from build123d import *

# Parameters (mm, degrees)
SKETCH1_W                      = 256.5
SKETCH1_H                      = 320
BASE_FLANGE1_DEPTH             = 0.9
EDGE_FLANGE1_STRIP_W           = 5.4
EDGE_FLANGE1_STRIP_H           = 0.9
EDGE_FLANGE1_STRIP_CUT_DEPTH   = 320
EDGE_FLANGE1_STRIP_2_W         = 5.4
EDGE_FLANGE1_STRIP_2_H         = 0.9
EDGE_FLANGE1_STRIP_CUT_2_DEPTH = 320
EDGE_FLANGE1_DEPTH             = 320
EDGE_FLANGE1_BEND_DEPTH        = 320
EDGE_FLANGE2_STRIP_W           = 5.4
EDGE_FLANGE2_STRIP_H           = 0.9
EDGE_FLANGE2_STRIP_CUT_DEPTH   = 320
EDGE_FLANGE2_DEPTH             = 320
CUT_EXTRUDE1_DEPTH             = 206.751482376


# Sheet-metal steps are written as plain solids
with BuildPart() as part:
    # Sketch1 → Base-Flange1 (new body)
    with BuildSketch(Plane.XY):
        Rectangle(SKETCH1_W, SKETCH1_H)
    extrude(amount=-BASE_FLANGE1_DEPTH)

    # Edge-Flange1 strip (across the edge) → Edge-Flange1 strip cut (cut)
    with BuildSketch(Plane(origin=(128.25, 160, -0.9), x_dir=(-1, 0, 0), z_dir=(0, -1, 0))):
        with Locations((-0.9, -0.45)):
            Rectangle(EDGE_FLANGE1_STRIP_W, EDGE_FLANGE1_STRIP_H)
    extrude(amount=EDGE_FLANGE1_STRIP_CUT_DEPTH, mode=Mode.SUBTRACT)

    # Edge-Flange1 strip 2 (across the edge) → Edge-Flange1 strip cut 2 (cut)
    with BuildSketch(Plane(origin=(-128.25, -160, -0.9), x_dir=(1, 0, 0), z_dir=(0, 1, 0))):
        with Locations((-0.9, -0.45)):
            Rectangle(EDGE_FLANGE1_STRIP_2_W, EDGE_FLANGE1_STRIP_2_H)
    extrude(amount=EDGE_FLANGE1_STRIP_CUT_2_DEPTH, mode=Mode.SUBTRACT)

    # Edge-Flange1 section (across the edge) → Edge-Flange1 (add)
    with BuildSketch(Plane(origin=(128.25, 160, -0.9), x_dir=(-1, 0, 0), z_dir=(0, -1, 0))):
        with BuildLine():
            Line((0, 0.9), (0, 15.1))
            Line((0, 15.1), (0.9, 15.1))
            Line((0.9, 15.1), (0.9, 0.9))
            ThreePointArc((0.9, 0.9), (1.163603897, 0.263603897), (1.8, 0))
            Line((1.8, 0), (1.8, -0.9))
            ThreePointArc((1.8, -0.9), (0.527207794, -0.372792206), (0, 0.9))
        make_face()
    extrude(amount=EDGE_FLANGE1_DEPTH)

    # Edge-Flange1 section 2 (across the edge) → Edge-Flange1 bend (add)
    with BuildSketch(Plane(origin=(-128.25, -160, -0.9), x_dir=(1, 0, 0), z_dir=(0, 1, 0))):
        with BuildLine():
            Line((0, 0.9), (0, 15.1))
            Line((0, 15.1), (0.9, 15.1))
            Line((0.9, 15.1), (0.9, 0.9))
            ThreePointArc((0.9, 0.9), (1.163603897, 0.263603897), (1.8, 0))
            Line((1.8, 0), (1.8, -0.9))
            ThreePointArc((1.8, -0.9), (0.527207794, -0.372792206), (0, 0.9))
        make_face()
    extrude(amount=EDGE_FLANGE1_BEND_DEPTH)

    # Edge-Flange2 strip (across the edge) → Edge-Flange2 strip cut (cut)
    with BuildSketch(Plane(origin=(127.35, 160, -16), x_dir=(0, 0, 1), z_dir=(0, -1, 0))):
        with Locations((-1.8, -0.45)):
            Rectangle(EDGE_FLANGE2_STRIP_W, EDGE_FLANGE2_STRIP_H)
    extrude(amount=EDGE_FLANGE2_STRIP_CUT_DEPTH, mode=Mode.SUBTRACT)

    # Edge-Flange2 section (across the edge) → Edge-Flange2 (add)
    with BuildSketch(Plane(origin=(127.35, 160, -16), x_dir=(0, 0, 1), z_dir=(0, -1, 0))):
        with BuildLine():
            Line((-0.9, 0.9), (-0.9, 14.1))
            Line((-0.9, 14.1), (0, 14.1))
            Line((0, 14.1), (0, 0.9))
            ThreePointArc((0, 0.9), (0.263603897, 0.263603897), (0.9, 0))
            Line((0.9, 0), (0.9, -0.9))
            ThreePointArc((0.9, -0.9), (-0.372792206, -0.372792206), (-0.9, 0.9))
        make_face()
    extrude(amount=EDGE_FLANGE2_DEPTH)

    # Sketch24 → Cut-Extrude1 (cut, through all)
    with BuildSketch(Plane.XY):
        with BuildLine():
            Line((101, 4.123105626), (101, -4.123105626))
            ThreePointArc((101, -4.123105626), (93, -9), (85, -4.123105626))
            Line((85, -4.123105626), (85, 4.123105626))
            ThreePointArc((85, 4.123105626), (93, 9), (101, 4.123105626))
        make_face()
    extrude(amount=-CUT_EXTRUDE1_DEPTH, mode=Mode.SUBTRACT)


solid = part.part
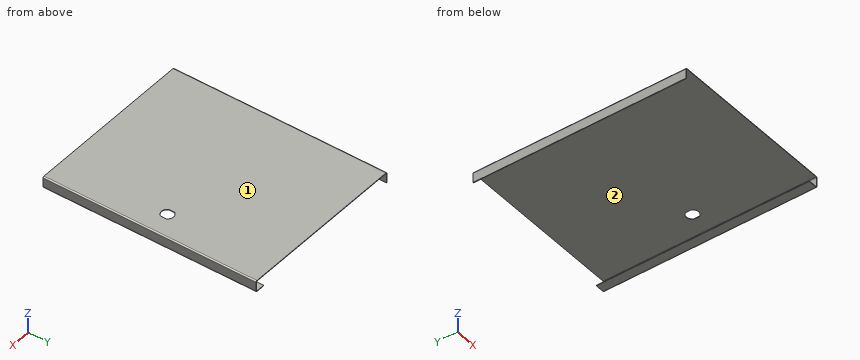
Input: part model. Units: mm. Frame: model coordinates. Face numbers are marked on the shaded views. Give positions to 0.01 mm unless a question says otherwise; leave off trailing zeros. Order: outer loops, then holes, each group sorted by start corner. A loop starts at its lowest first (then second) coordinate and runs counter-clockwise, first axis right, second up. Notation, with made-up numbers: M 21,14.25 L 36,14.25 A11 cw 36,21.25 Z; hole C 61.25,-34 d6. An arc over 180 degrees is marked long. Answer as a JSON object with one key per item and string values.
1. Pull-direction query (X, two-part tool) for the marked faces 1 and 2; classes: +X half, -X half, draft (parallel to the pull), parting line (faces both ways), or undercut.
Result sheet:
{"face 1": "draft", "face 2": "undercut"}
2. Cut plane A-A, the plane z = -11.5. Output: boundary loops of the cut face in (x, y).
Result sheet:
{"outline": "M -128.25,-160 L -127.35,-160 L -127.35,160 L -128.25,160 Z; M 127.35,-160 L 128.25,-160 L 128.25,160 L 127.35,160 Z"}
3. Ray query, line 1 (X direction, y = 112, z = -7); line 2 (Z direction, x = -10.5, y = 62). Return the intervals inside material, ascending. Write a range as [from, to].
Result sheet:
{"line 1": "[-128.25, -127.35], [127.35, 128.25]", "line 2": "[-0.9, 0]"}
4. Cut plane B-B, the plane y = 55.5. Output: boundary loops of the cut face in (x, z), and give its area (3 significant figures).
Result sheet:
{"outline": "M -128.25,-16 L -127.35,-16 L -127.35,-1.8 A0.9 cw -126.45,-0.9 L 126.45,-0.9 A0.9 cw 127.35,-1.8 L 127.35,-15.1 A0.9 cw 126.45,-16 L 113.25,-16 L 113.25,-16.9 L 126.45,-16.9 A1.8 ccw 128.25,-15.1 L 128.25,-1.8 A1.8 ccw 126.45,0 L -126.45,0 A1.8 ccw -128.25,-1.8 Z", "area": "270 mm²"}
5. Cut plane C-C, the plane x = -15.5. Output: boundary loops of the cut face in (y, z).
Result sheet:
{"outline": "M -160,-0.9 L 160,-0.9 L 160,0 L -160,0 Z"}
6. First-contact query: P1, Ø1, axis at x = -47, z = -2, coming from the +Y side; P2, Ø0.7, axis at y = -0.5, z = -0.5, coming from the +X side; P3, Ø0.5, axis at x = -128, y = 54.5, coming from the -Z side; P4, Ø1, axis at y = -0.5, z = -0.5, coming from the -X side. Flat tips, straight axial feed; report the tip coordinate or a pass-through.
Result sheet:
{"P1": "through", "P2": "x = 127.98", "P3": "z = -16", "P4": "x = -128.06"}
